Read the model definition and answer for the solid it produces. Units are mm, in the model's axes. A direction names the side the tool comes from. Coordinates: 2 decimals unless noted, no trailing zeros. Loops run counter-clockwise (first coordinate to the right, second up) from the corner with the lowest first, then second, coordinate; pieces in that order, holes last. Notation, with made-up numbers: M -10,-29.75 L 0,-29.75 A8 ccw 0,-17.75 Z; hole C -15.5,76.5 d2. An arc over 180 degrees is marked long. Put each result on its own line as item: value.
from build123d import *

# Parameters (mm, degrees)
F0_R           = 20
F0_R_2         = 25
F1_DEPTH       = 10
F2_R           = 23.5
F2_R_2         = 20
F2_R_3         = 28.5
F2_R_4         = 25
F3_DEPTH       = 3
F4_D           = 3
F4_CSINK_D     = 10
F4_CSINK_ANGLE = 90


with BuildPart() as f1:
    # F0 (on Top) → F1 (new body)
    with BuildSketch(Plane.XY):
        with BuildLine():
            Line((98.5, 105), (-128.5, 105))
            ThreePointArc((-128.5, 105), (-133.096194, 103.096194), (-135, 98.5))
            Line((-135, 98.5), (-135, -98.5))
            ThreePointArc((-135, -98.5), (-133.096194, -103.096194), (-128.5, -105))
            Line((-128.5, -105), (98.5, -105))
            ThreePointArc((98.5, -105), (103.096194, -103.096194), (105, -98.5))
            Line((105, -98.5), (105, 98.5))
            ThreePointArc((105, 98.5), (103.096194, 103.096194), (98.5, 105))
        make_face()
        with Locations((-100, 0)):
            Circle(F0_R, mode=Mode.SUBTRACT)
        Circle(F0_R_2, mode=Mode.SUBTRACT)
    extrude(amount=-F1_DEPTH)

    # F2 (on face) → F3 (cut)
    with BuildSketch(Plane.XY):
        with Locations((-100, 0)):
            Circle(F2_R)
        with Locations((-100, 0)):
            Circle(F2_R_2, mode=Mode.SUBTRACT)
        Circle(F2_R_3)
        Circle(F2_R_4, mode=Mode.SUBTRACT)
    extrude(amount=-F3_DEPTH, mode=Mode.SUBTRACT)

    # F4 (through all)
    with Locations(Plane.XY):
        with Locations((-115, 85), (85, 85), (85, -85), (-115, -85)):
            CounterSinkHole(F4_D / 2, F4_CSINK_D / 2, counter_sink_angle=F4_CSINK_ANGLE)


solid = f1.part
1) Which of the six approach directions +Z, -Z, +X, -X, +Y, -Y give full straight-line access (tool end or side, diameter ignored) to faces 1 (the cylindrical face through (103.045, -103.146, -4.93)), 2 (the cylindrical face through (26.327, -10.916, -1.479))?
Answer list:
face 1: +Z, -Z, +X, -Y
face 2: +Z
2) Find section C-C, the plane z = -1.5. Write down the section's boundary in (x, y).
Answer list:
outline: M -135,-98.5 A6.5 ccw -128.5,-105 L 98.5,-105 A6.5 ccw 105,-98.5 L 105,98.5 A6.5 ccw 98.5,105 L -128.5,105 A6.5 ccw -135,98.5 Z; hole C -100,0 d47; hole C -115,-85 d7; hole C -115,85 d7; hole C 0,0 d57; hole C 85,-85 d7; hole C 85,85 d7
3) Determine the mould class of faces 3 (the cylindrical face through (-133.045, 103.146, -4.93)), 4 (the flat face through (-17, 25, 0)), 5 (the flat face through (-93, 19, -3)) for opening direction X: released by +X, released by -X, zero draft, split by the parting line, or undercut.
Answer list:
face 3: released by -X
face 4: zero draft
face 5: undercut
4) Find section A-A, the plane y = 0. Write down the section's boundary in (x, z).
Answer list:
outline: M -135,-10 L -120,-10 L -120,-3 L -123.5,-3 L -123.5,0 L -135,0 Z; M -80,-10 L -25,-10 L -25,-3 L -28.5,-3 L -28.5,0 L -76.5,0 L -76.5,-3 L -80,-3 Z; M 25,-10 L 105,-10 L 105,0 L 28.5,0 L 28.5,-3 L 25,-3 Z
5) Straight lines are drawn through the part: line 1 (X direction, y = -85, z = -4.75); line 2 (Y direction, x = 0, z = -7.75); line 3 (X direction, y = 17, z = -3.75). For each, find the intervals that lie inside material, in ascending order. Write a range as [from, to].
Answer list:
line 1: x = [-135, -116.5], [-113.5, 83.5], [86.5, 105]
line 2: y = [-105, -25], [25, 105]
line 3: x = [-135, -110.54], [-89.46, -18.33], [18.33, 105]
6) Find section B-B, the plane x = 0. Write down the section's boundary in (y, z).
Answer list:
outline: M -105,-10 L -25,-10 L -25,-3 L -28.5,-3 L -28.5,0 L -105,0 Z; M 25,-10 L 105,-10 L 105,0 L 28.5,0 L 28.5,-3 L 25,-3 Z
